```python
from build123d import *

# Parameters (mm, degrees)
SKETCH1_R           = 1
BOSS_EXTRUDE1_DEPTH = 1.5


with BuildPart() as part:
    # Sketch1 → Boss-Extrude1 (new body)
    with BuildSketch(Plane.XY):
        with BuildLine():
            ThreePointArc((0, 3.458652708), (-10.55, -7.091347292), (0, -17.641347292))
            ThreePointArc((0, -17.641347292), (4.45, -22.091347292), (0, -26.541347292))
            ThreePointArc((0, -26.541347292), (-2.05, -28.591347292), (0, -30.641347292))
            ThreePointArc((0, -30.641347292), (8.55, -22.091347292), (0, -13.541347292))
            ThreePointArc((0, -13.541347292), (-6.45, -7.091347292), (0, -0.641347292))
            ThreePointArc((0, -0.641347292), (2.05, 1.408652708), (0, 3.458652708))
        make_face()
        with Locations((0, 1.408652708)):
            Circle(SKETCH1_R, mode=Mode.SUBTRACT)
        with Locations((0, -28.591347292)):
            Circle(SKETCH1_R, mode=Mode.SUBTRACT)
    extrude(amount=BOSS_EXTRUDE1_DEPTH)


solid = part.part
```
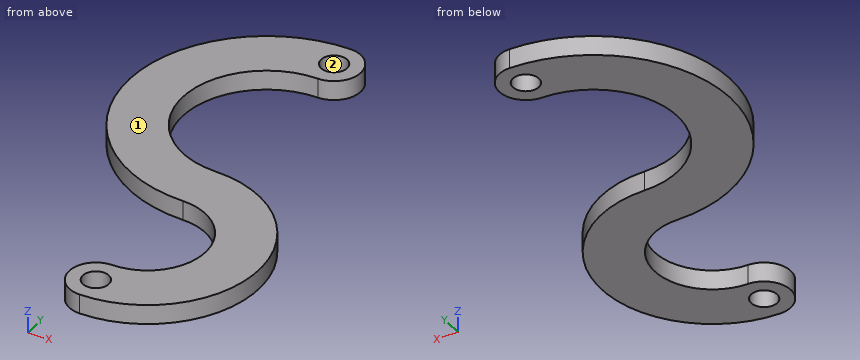
CAD build for the part. Positions are in the model's coordinates, mm. Face numbers are marked on the shaded views. Give positions to 0.01 mm unless a question says otherwise; leave off trailing zeros. Write each loop counter-clockwise with the first axis right and the second up, starting at its lowest first coordinate (ties: lowest second). Pieces come first, ordered by that corner, then holes. Notation, with made-up numbers: M 24.5,-7.5 L 63.5,-7.5 A21 ccw 63.5,6.5 Z; hole C 86,-3.75 d7. An arc over 180 degrees is marked long. Return JSON: item names as keys, results as strings. Group by question number.
(1) Drill centre lines: L1, parallel to Y at x = 1.75, z = 0.35; L2, parallel to Y at x = -0.75, z = 0.4; L3, parallel to X at y = -22.5, z = 1.1. Where is each one in solid material? Low to high. Write a range as [from, to].
(2) Band-saw the part on A-A (x = 2.5). Give the cut face in (y, z) (3 decimals).
(3) Band-saw the part on C-C (z = 0.3). Give the cut face in (x, y).
(4) Band-saw the part on B-B (y = 1). Give the cut face in (x, z), and give its area (3 significant figures).
(5) Mould opens along Y. For the marked faces 1 and 2 say: pulls with the +Y half, pulls with the -Y half, needs draft (parallel to the pull), parting line crosses it, or undercut.
(6) Band-saw the part on D-D (x = -8.75). Give the cut face in (y, z).
Entries:
{
 "1": {"L1": "y = [-30.46, -26.18], [-18, -13.72], [0.34, 2.48]", "L2": "y = [-30.5, -29.25], [-27.93, -26.68], [-17.61, -13.5], [-0.69, 0.75], [2.07, 3.43]", "L3": "x = [4.43, 8.54]"},
 "2": {"outline": "M -30.268,0 L -25.773,0 L -25.773,1.5 L -30.268,1.5 Z; M -18.41,0 L -13.915,0 L -13.915,1.5 L -18.41,1.5 Z"},
 "3": {"outline": "M 0,-30.64 A8.55 ccw 0,-13.54 A6.45 cw 0,-0.64 A2.05 ccw 0,3.46 A10.55 ccw 0,-17.64 A4.45 cw 0,-26.54 A2.05 ccw Z; hole C 0,-28.59 d2; hole C 0,1.41 d2"},
 "4": {"outline": "M -6.77,0 L -0.91,0 L -0.91,1.5 L -6.77,1.5 Z; M 0.91,0 L 2.01,0 L 2.01,1.5 L 0.91,1.5 Z", "area": "10.4 mm^2"},
 "5": {"face 1": "needs draft", "face 2": "undercut"},
 "6": {"outline": "M -12.99,0 L -1.2,0 L -1.2,1.5 L -12.99,1.5 Z"}
}
